from build123d import *

# Parameters (mm, degrees)
ESBO_O1_W                = 8
ESBO_O1_H                = 21.6
RESSALTO_EXTRUS_O1_DEPTH = 2
ESBO_O2_W                = 8
ESBO_O2_H                = 2.5
RESSALTO_EXTRUS_O2_DEPTH = 8
ESBO_O3_R                = 1.6
CORTE_EXTRUS_O1_DEPTH    = 8
FILETE1_R                = 2
FILETE2_R                = 2
FILETE3_R                = 1
FILETE4_R                = 1
CHANFRO1_SIZE            = 1
FILETE5_R                = 0.5
FILETE6_R                = 0.5
FILETE7_R                = 0.5
FILETE8_R                = 0.5
FILETE9_R                = 0.5
FILETE10_R               = 0.5


with BuildPart() as part:
    # Esboço1 → Ressalto-extrusão1 (new body)
    with BuildSketch(Plane(origin=(0, 0, 0), x_dir=(1, 0, 0), z_dir=(0, 1, 0))):
        Rectangle(ESBO_O1_W, ESBO_O1_H)
    extrude(amount=RESSALTO_EXTRUS_O1_DEPTH)

    # Esboço2 → Ressalto-extrusão2 (add)
    with BuildSketch(Plane(origin=(0, 2, 0), x_dir=(1, 0, 0), z_dir=(0, 1, 0))):
        with Locations((0, -9.55)):
            Rectangle(ESBO_O2_W, ESBO_O2_H)
        with Locations((0, -0.45)):
            Rectangle(ESBO_O2_W, ESBO_O2_H)
    extrude(amount=RESSALTO_EXTRUS_O2_DEPTH)

    # Esboço3 → Corte-extrusão1 (cut)
    with BuildSketch(Plane(origin=(0, 2, 0), x_dir=(1, 0, 0), z_dir=(0, 1, 0))):
        with Locations(Location((0, 6.8, 0), (0, 0, 270))):
            Circle(ESBO_O3_R)
    extrude(amount=-CORTE_EXTRUS_O1_DEPTH, mode=Mode.SUBTRACT)

    # Filete1
    filete1_edges = [part.edges().sort_by_distance(p)[0] for p in [
        (-4, 1, -10.8),
    ]]
    fillet(filete1_edges, radius=FILETE1_R)

    # Filete2
    filete2_edges = [part.edges().sort_by_distance(p)[0] for p in [
        (4, 1, -10.8),
    ]]
    fillet(filete2_edges, radius=FILETE2_R)

    # Filete3
    filete3_edges = [part.edges().sort_by_distance(p)[0] for p in [
        (4, 5, 10.8),
    ]]
    fillet(filete3_edges, radius=FILETE3_R)

    # Filete4
    filete4_edges = [part.edges().sort_by_distance(p)[0] for p in [
        (-4, 5, 10.8),
    ]]
    fillet(filete4_edges, radius=FILETE4_R)

    # Chanfro1
    chanfro1_edges = [part.edges().sort_by_distance(p)[0] for p in [
        (0, 2, -0.8),
    ]]
    chamfer(chanfro1_edges, length=CHANFRO1_SIZE)

    # Filete5
    filete5_edges = [part.edges().sort_by_distance(p)[0] for p in [
        (4, 6.5, -0.8),
    ]]
    fillet(filete5_edges, radius=FILETE5_R)

    # Filete6
    filete6_edges = [part.edges().sort_by_distance(p)[0] for p in [
        (-4, 6.5, -0.8),
    ]]
    fillet(filete6_edges, radius=FILETE6_R)

    # Filete7
    filete7_edges = [part.edges().sort_by_distance(p)[0] for p in [
        (4, 6, 8.3),
    ]]
    fillet(filete7_edges, radius=FILETE7_R)

    # Filete8
    filete8_edges = [part.edges().sort_by_distance(p)[0] for p in [
        (-4, 6, 8.3),
    ]]
    fillet(filete8_edges, radius=FILETE8_R)

    # Filete9
    filete9_edges = [part.edges().sort_by_distance(p)[0] for p in [
        (-4, 6, 1.7),
    ]]
    fillet(filete9_edges, radius=FILETE9_R)

    # Filete10
    filete10_edges = [part.edges().sort_by_distance(p)[0] for p in [
        (4, 6, 1.7),
    ]]
    fillet(filete10_edges, radius=FILETE10_R)


solid = part.part
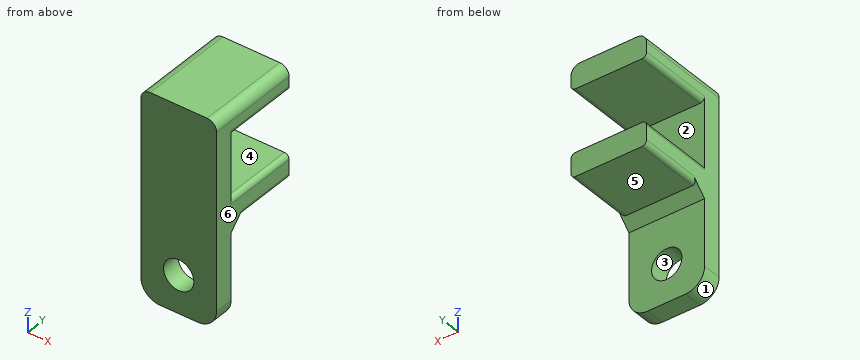
Input: part model. Units: mm. Frame: model coordinates. Face numbers are marked on the shaded views. A direction names the side the tool comes from. Coordinates: 2 decimals unless noted, no trailing zeros. Order: outer loops, then holes, each group sorted by start corner. A loop starts at its lowest first (then second) coordinate and runs counter-clockwise, first axis right, second up. Notation, with made-up numbers: M 26,83.5 L 50,83.5 A26 ccw 50,116.5 Z; hole C 51.25,70.5 d6. An arc over 180 degrees is marked long. Answer in a Markdown table with one row per item.
(1) Section query D-D, the plane x = 0. Output: boundary loops of the cut face in (y, z).
Numbers:
| item | result |
|---|---|
| outline | M 0,-10.8 L 2,-10.8 L 2,-8.4 L 0,-8.4 Z; M 0,-5.2 L 2,-5.2 L 2,-1.8 L 3,-0.8 L 10,-0.8 L 10,1.7 L 2,1.7 L 2,8.3 L 10,8.3 L 10,10.8 L 0,10.8 Z |
(2) Section query C-C, the plane y = 1. Output: boundary loops of the cut face in (x, z).
Numbers:
| item | result |
|---|---|
| outline | M -4,-8.8 A2 ccw -2,-10.8 L 2,-10.8 A2 ccw 4,-8.8 L 4,9.8 A1 ccw 3,10.8 L -3,10.8 A1 ccw -4,9.8 Z; hole C 0,-6.8 d3.2 |
(3) Access query for the marked faces 4, 5 and 6. Directions: +Z, -Z, +X, -X, +Y, -Y. A direction counts if a zero-diameter tool reaches every point of the face in a straight line with its end or side. Return the directions, or none.
Numbers:
| item | result |
|---|---|
| face 4 | +X, -X, +Y |
| face 5 | -Z, +X, -X, +Y |
| face 6 | +Z, -Z, +X, +Y, -Y |
(4) Section query B-B, the plane z = -6.8. Output: boundary loops of the cut face in (x, y), plus the area to 3 significant figures.
Numbers:
| item | result |
|---|---|
| outline | M -4,0 L -1.6,0 L -1.6,2 L -4,2 Z; M 1.6,0 L 4,0 L 4,2 L 1.6,2 Z |
| area | 9.60 mm^2 |
(5) Section query A-A, the plane y = 2.5. Output: boundary loops of the cut face in (x, z).
Numbers:
| item | result |
|---|---|
| outline | M -4,-1.3 L 4,-1.3 L 4,1.2 A0.5 ccw 3.5,1.7 L -3.5,1.7 A0.5 ccw -4,1.2 Z; M -4,8.8 A0.5 ccw -3.5,8.3 L 3.5,8.3 A0.5 ccw 4,8.8 L 4,9.8 A1 ccw 3,10.8 L -3,10.8 A1 ccw -4,9.8 Z |
(6) Contact query for flat-ended pins moving along their axis: pin 1 Ø3 at (x, z) = (0, -6.8) entering from +Y; pin 2 Ø2 at (x, y) = (0, 5.5) entering from -Z. Output: stop coordinate, or through.
Numbers:
| item | result |
|---|---|
| pin 1 | passes through |
| pin 2 | stops at z = -0.8 |
(7) Draft query along X for the marked faces 1, 2 and 3. Return one class per face: pulls with the +X half, pulls with the -X half, needs draft (parallel to the pull), parting line crosses it, or undercut.
Numbers:
| item | result |
|---|---|
| face 1 | pulls with the -X half |
| face 2 | needs draft |
| face 3 | undercut |
(8) Material intervals for line 1 (Z direction, x = 1.75, y = 3.5); line 2 (X direction, y = 1.3, z = -6.8); line 3 (Z direction, x = 1.25, y = 2.5), sorted ascending. Write a range as [from, to].
Numbers:
| item | result |
|---|---|
| line 1 | z = [-0.8, 1.7], [8.3, 10.8] |
| line 2 | x = [-4, -1.6], [1.6, 4] |
| line 3 | z = [-1.3, 1.7], [8.3, 10.8] |
